Here's how the part is built. I have some questions about the finished solid (model axes, mm). Face numbers are marked on the shaded views. A direction names the side the tool comes from. Give positions to 0.01 mm unless a question says otherwise; leave off trailing zeros. Loops run counter-clockwise (first coordinate to the right, second up) from the corner with the lowest first, then second, coordinate; pieces in that order, holes last. Notation, with made-up numbers: (-21, 80) -> (-2, 80) arc R25 cw to (-2, 103) -> close; hole circle Ø10 at (-32, -39). An arc over 180 degrees is marked (long way). Answer in a Markdown table with one row per item. Add a question column.
Item 1: For P1, Ø3, axis at x = 43, z = 11, coming from the -Y side; P2, Ø2, axis at x = 17.31, z = 17.86, coming from the -Y side; P3, Ø8, axis at x = 16.5, z = 7, coming from the +Y side, each with a flat end and sliding along its axis, tell me the tip position at first contact or that it passes through.
Item 2: Which directions (+Z, -Z, +X, -X, +Y, -Y) give clear straight access to the entire face, cutting with the end or side of a thin tool? Please do the marked faces 1, 2, 3 and 4.
Item 3: If we section it at C-C (y = 36): Write out the boundary of the cut face in (x, z).
Item 4: If we section it at B-B (z = 9.93): Write out the boundary of the cut face in (x, y), then the cut area to 3 significant figures.
Item 5: If we section it at D-D (z = 5.75): Write out the boundary of the cut face in (x, y), then the cut area to 3 significant figures.
Item 6: If I drill on line 1 (X direction, y = 1, z = 17.75); line 2 (Z direction, x = 38, y = 1); line 3 (Y direction, x = 9, z = 12.5), over which ranges is the centre line in solid material (lowest first)?
Item 7: If we section it at A-A (x = 38.43): Write out the boundary of the cut face in (y, z).
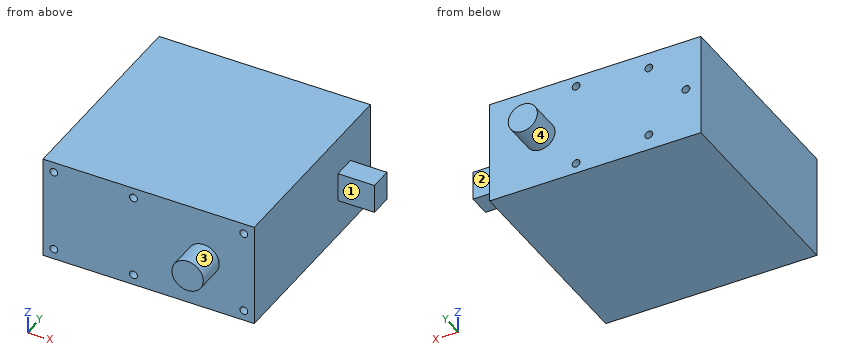
```python
from build123d import *

# Parameters (mm, degrees)
SKETCH1_W              = 40.43
SKETCH1_H              = 40.16
SERVOBODY_DEPTH        = 19.86
SKETCH2_R              = 2.79
GEARHINGE_DEPTH        = 6.1
SKETCH3_R              = 3.01
SMOOTHHINGE_DEPTH      = 5.5
SKETCH4_R              = 0.75
GEARSCREWHOLES_DEPTH   = 2
SKETCH5_R              = 0.75
SMOOTHSCREWHOLES_DEPTH = 2
SKETCH6_W              = 5.54
SKETCH6_H              = 4.32
CABLE_DEPTH            = 7


with BuildPart() as part:
    # Sketch1 → ServoBody (new body)
    with BuildSketch(Plane.XY):
        with Locations((20.215, 20.08)):
            Rectangle(SKETCH1_W, SKETCH1_H)
    extrude(amount=SERVOBODY_DEPTH)

    # Sketch2 → GearHinge (add)
    with BuildSketch(Plane(origin=(0, 40.16, 0), x_dir=(1, 0, 0), z_dir=(0, 1, 0))):
        with Locations(Location((30.71, -9.93, 0), (0, 0, 90))):
            Circle(SKETCH2_R)
    extrude(amount=GEARHINGE_DEPTH)

    # Sketch3 → SmoothHinge (add)
    with BuildSketch(Plane.XZ):
        with Locations(Location((30.71, 9.93, 0), (0, 0, 90))):
            Circle(SKETCH3_R)
    extrude(amount=SMOOTHHINGE_DEPTH)

    # Sketch4 → GearScrewHoles (cut)
    with BuildSketch(Plane(origin=(0, 40.16, 0), x_dir=(1, 0, 0), z_dir=(0, 1, 0))):
        with Locations(Location((23.88, -1.98, 0), (0, 0, 270))):
            Circle(SKETCH4_R)
        with Locations(Location((23.88, -17.88, 0), (0, 0, 270))):
            Circle(SKETCH4_R)
        with Locations(Location((2.87, -9.93, 0), (0, 0, 270))):
            Circle(SKETCH4_R)
        with Locations(Location((9.96, -3.05, 0), (0, 0, 270))):
            Circle(SKETCH4_R)
        with Locations(Location((9.96, -16.81, 0), (0, 0, 270))):
            Circle(SKETCH4_R)
    extrude(amount=-GEARSCREWHOLES_DEPTH, mode=Mode.SUBTRACT)

    # Sketch5 → SmoothScrewHoles (cut)
    with BuildSketch(Plane.XZ):
        with Locations(Location((17.31, 17.86, 0), (0, 0, 270))):
            Circle(SKETCH5_R)
        with Locations(Location((38.43, 17.86, 0), (0, 0, 270))):
            Circle(SKETCH5_R)
        with Locations(Location((2.07, 17.86, 0), (0, 0, 270))):
            Circle(SKETCH5_R)
        with Locations(Location((17.31, 2, 0), (0, 0, 270))):
            Circle(SKETCH5_R)
        with Locations(Location((38.43, 2, 0), (0, 0, 270))):
            Circle(SKETCH5_R)
        with Locations(Location((2.07, 2, 0), (0, 0, 270))):
            Circle(SKETCH5_R)
    extrude(amount=-SMOOTHSCREWHOLES_DEPTH, mode=Mode.SUBTRACT)

    # Sketch6 → Cable (add)
    with BuildSketch(Plane(origin=(40.43, 0, 0), x_dir=(0, 0, -1), z_dir=(1, 0, 0))):
        with Locations((-9.93, 31.1)):
            Rectangle(SKETCH6_W, SKETCH6_H)
    extrude(amount=CABLE_DEPTH)


solid = part.part
```
Recorded:
| question | item | result |
|---|---|---|
| 1 | P1 | stops at y = 28.94 |
| 1 | P2 | stops at y = 0 |
| 1 | P3 | stops at y = 40.16 |
| 2 | face 1 | +Z, -Z, +X, -Y |
| 2 | face 2 | +Z, -Z, +X, +Y |
| 2 | face 3 | -Y |
| 2 | face 4 | +Y |
| 3 | outline | (0, 0) -> (40.43, 0) -> (40.43, 19.86) -> (0, 19.86) -> close |
| 4 | outline | (0, 0) -> (27.7, 0) -> (27.7, -5.5) -> (33.72, -5.5) -> (33.72, 0) -> (40.43, 0) -> (40.43, 28.94) -> (47.43, 28.94) -> (47.43, 33.26) -> (40.43, 33.26) -> (40.43, 40.16) -> (33.5, 40.16) -> (33.5, 46.26) -> (27.92, 46.26) -> (27.92, 40.16) -> (3.62, 40.16) -> (3.62, 38.16) -> (2.12, 38.16) -> (2.12, 40.16) -> (0, 40.16) -> close |
| 4 | area | 1,720 mm^2 |
| 5 | outline | (0, 0) -> (40.43, 0) -> (40.43, 40.16) -> (0, 40.16) -> close |
| 5 | area | 1,620 mm^2 |
| 6 | line 1 | x = 0 to 1.33, 2.81 to 16.57, 18.05 to 37.69, 39.17 to 40.43 |
| 6 | line 2 | z = 0 to 1.39, 2.61 to 17.25, 18.47 to 19.86 |
| 6 | line 3 | y = 0 to 40.16 |
| 7 | outline | (0, 0) -> (40.16, 0) -> (40.16, 19.86) -> (0, 19.86) -> (0, 18.61) -> (2, 18.61) -> (2, 17.11) -> (0, 17.11) -> (0, 2.75) -> (2, 2.75) -> (2, 1.25) -> (0, 1.25) -> close |
